For this review, take the finished solid that the model builds, in its own axes (mm). A direction names the side the tool comes from. Round coordinates to 2 decimals unless told otherwise and drop trailing zeros. Write each loop counter-clockwise with the first axis right and the second up, starting at its lowest first coordinate (ties: lowest second). Pieces come first, ordered by that corner, then holes. Notation, with made-up numbers: (55.5, -17) -> (92.5, -17) arc R26 cw to (92.5, 2) -> close; hole circle Ø8 at (-7, -3). An arc over 180 degrees is marked (long way). Write each question's results on one line, items separated by ' | '. Start each with the question number.
Item 1: Tool access review of faces 1 (the flat face through (165.1, 13, 24)), 2 (the flat face through (0, 2, 13)), 3 (the flat face through (19.05, 13, 24)): name each direction out of +Z, -Z, +X, -X, +Y, -Y from which nothing blocks a thin tool from reaching the whole face with its end or side.
Item 2: To check wall thickness, follow line 1 along Y through (x, z) = (117.5, 21.75); line 2 along X through (y, z) = (8.5, 23.5). State the ranges of each line that lie inside material, in increasing order.
Item 3: Add section A-A (z = 18.5). State the section outline as (x, y) points, plus the area to 3 significant figures.
Item 4: Clearance check with flat-ended pins moving along their axes: pin 1 (12 mm diameter, centred on y = 14, z = 16.5, fed in from -X); pin 2 (4 mm diameter, centred on x = 104, y = 4.5, fed in from -Z); pin 3 (3.5 mm diameter, centred on y = 15.5, z = 2, fed in from +X). State where each tip first meets the part, or that it passes through.
Item 5: The part is to be moulded in two halves that separate along Z. For faces 4 (the flat face through (91, 13, 3.048)), 5 (the flat face through (91, 13, 22.352)), 6 (the flat face through (184.15, 2, 13)), 7 (the flat face through (91, 13, 0)), say which applies: +Z half, -Z half, draft (parallel to the pull), parting line (faces both ways), or undercut.
Item 6: Add section B-B (y = 15.25). State the section outline as (x, z) points.
Item 7: Add section C-C (x = 124). State the section outline as (y, z) points, plus the area to 3 significant figures.
from build123d import *

# Parameters (mm, degrees)
SKETCH1_W           = 19.304
SKETCH1_H           = 19.304
BOSS_EXTRUDE1_DEPTH = 184.15
SKETCH2_W           = 25.4
SKETCH2_H           = 19.304
CUT_EXTRUDE1_DEPTH  = 19.05
SKETCH3_W           = 25.4
SKETCH3_H           = 19.304
CUT_EXTRUDE2_DEPTH  = 19.05


with BuildPart() as part:
    # Sketch1 → Boss-Extrude1 (new body)
    with BuildSketch(Plane(origin=(0, 0, 0), x_dir=(0, 0, -1), z_dir=(1, 0, 0))):
        with BuildLine():
            Line((0, 2.54), (0, 22.86))
            ThreePointArc((0, 22.86), (-0.743948776, 24.656051224), (-2.54, 25.4))
            Line((-2.54, 25.4), (-22.86, 25.4))
            ThreePointArc((-22.86, 25.4), (-24.656051224, 24.656051224), (-25.4, 22.86))
            Line((-25.4, 22.86), (-25.4, 2.54))
            ThreePointArc((-25.4, 2.54), (-24.656051224, 0.743948776), (-22.86, 0))
            Line((-22.86, 0), (-2.54, 0))
            ThreePointArc((-2.54, 0), (-0.743948776, 0.743948776), (0, 2.54))
        make_face()
        with Locations((-12.7, 12.7)):
            Rectangle(SKETCH1_W, SKETCH1_H, mode=Mode.SUBTRACT)
    extrude(amount=BOSS_EXTRUDE1_DEPTH)

    # Sketch2 → Cut-Extrude1 (cut)
    with BuildSketch(Plane(origin=(184.15, 0, 0), x_dir=(0, 0, -1), z_dir=(1, 0, 0))):
        with Locations((-12.7, 12.7)):
            Rectangle(SKETCH2_W, SKETCH2_H)
    extrude(amount=-CUT_EXTRUDE1_DEPTH, mode=Mode.SUBTRACT)

    # Sketch3 → Cut-Extrude2 (cut)
    with BuildSketch(Plane.ZY):
        with Locations((12.7, 12.7)):
            Rectangle(SKETCH3_W, SKETCH3_H)
    extrude(amount=-CUT_EXTRUDE2_DEPTH, mode=Mode.SUBTRACT)


solid = part.part
Responses:
1) face 1: +Z, -Z, +X | face 2: +Z, -Z, -X, +Y, -Y | face 3: +Z, -Z, -X
2) line 1: y = 0 to 3.05, 22.35 to 25.4 | line 2: x = 19.05 to 165.1
3) outline: (0, 0) -> (184.15, 0) -> (184.15, 3.05) -> (0, 3.05) -> close; (0, 22.35) -> (184.15, 22.35) -> (184.15, 25.4) -> (0, 25.4) -> close | area: 1,120 mm^2
4) pin 1: stops at x = 19.05 | pin 2: stops at z = 0 | pin 3: stops at x = 165.1
5) face 4: undercut | face 5: undercut | face 6: draft | face 7: -Z half
6) outline: (19.05, 0) -> (165.1, 0) -> (165.1, 3.05) -> (19.05, 3.05) -> close; (19.05, 22.35) -> (165.1, 22.35) -> (165.1, 25.4) -> (19.05, 25.4) -> close
7) outline: (0, 2.54) arc R2.54 ccw to (2.54, 0) -> (22.86, 0) arc R2.54 ccw to (25.4, 2.54) -> (25.4, 22.86) arc R2.54 ccw to (22.86, 25.4) -> (2.54, 25.4) arc R2.54 ccw to (0, 22.86) -> close; hole (3.05, 3.05) -> (22.35, 3.05) -> (22.35, 22.35) -> (3.05, 22.35) -> close | area: 267 mm^2
